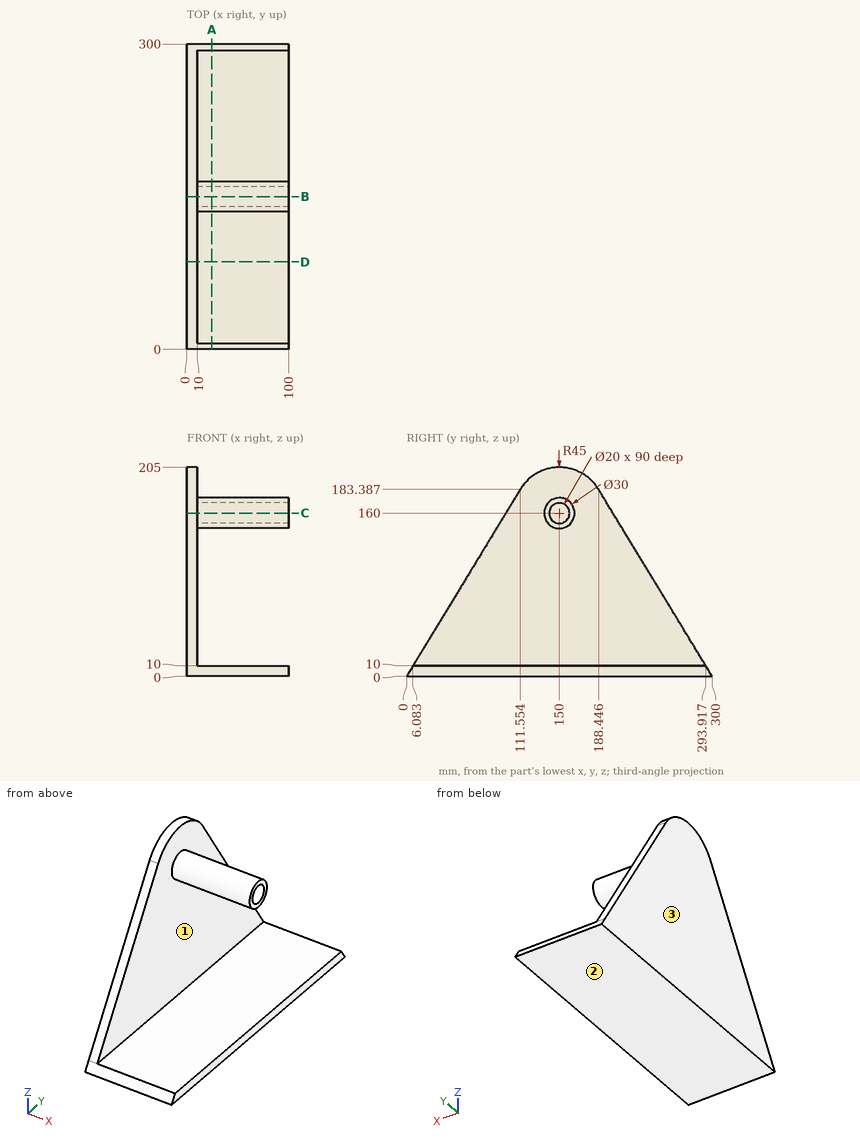
Input: dimensioned drawing with shaded views. Units: mm. Origin: part minimum x, y, z. Coordinates: 2 decimals unless noted, no trailing zeros. Loops run counter-clockwise (first coordinate to the right, second up) from the corner with the lowest first, then second, coordinate; pieces in that order, holes last. Notation, with made-up numbers: (32, 75) -> (39, 75) arc R21 ccw to (39, 112) -> close; hole circle Ø4 at (37, 31). An arc over 180 degrees is marked (long way). One line per item, written item: value. Start each with the question number.
Q1. Line query: line 1 along Z through (x, y) = (53, 150); line 2 along X through (y, z) = (30.5, 28); line 3 along Y through (x, z) = (70.5, 151) (1 decimal). Output: solid intervals per line, ascending.
Q2. Contact query for flat-ended pins moving along their axis: P1, Ø4, axis at x = 21, y = 85.5, coming from the +Z side; P2, Ø1.5, axis at x = 30.5, z = 166.5, coming from the +Y side (1 decimal); P3, Ø1, axis at x = 54.5, z = 156.5, coming from the +Y side. Output: stop coordinate, or through.
Q3. Mould query, pull axis Z, two halves, no side actions, for the marked faces 1, 2 and 3. Classes: pulls with the +Z half, pulls with the -Z half, needs draft (parallel to the pull), parting line crosses it, or undercut.
Q4. Section query A-A, the plane x = 24.5. Return the cut outline in (y, z), and give its area (3 significant figures).
Q5. Section query D-D, the plane y = 86. Return the cut outline in (x, z), and give its area (3 significant figures).
Q6. Section query C-C, the plane z = 160. Return the cut outline in (x, y).
Q7. Section query B-B, the plane y = 150. Return the cut outline in (x, z), and give its area (3 significant figures).
Results:
1. line 1: 0 to 10, 145 to 150, 170 to 175
1. line 2: 0 to 10
1. line 3: 138 to 145.6, 154.4 to 162
2. P1: z = 10
2. P2: y = 163.9
2. P3: y = 164.7
3. face 1: undercut
3. face 2: pulls with the -Z half
3. face 3: needs draft
4. outline: (0, 0) -> (300, 0) -> (293.92, 10) -> (6.08, 10) -> close; circle Ø30 at (150, 160); hole circle Ø20 at (150, 160)
4. area: 3,330 mm^2
5. outline: (0, 0) -> (100, 0) -> (100, 10) -> (10, 10) -> (10, 141.38) -> (0, 141.38) -> close
5. area: 2,310 mm^2
6. outline: (0, 97.33) -> (10, 97.33) -> (10, 135) -> (100, 135) -> (100, 140) -> (10, 140) -> (10, 160) -> (100, 160) -> (100, 165) -> (10, 165) -> (10, 202.67) -> (0, 202.67) -> close
7. outline: (0, 0) -> (100, 0) -> (100, 10) -> (10, 10) -> (10, 145) -> (100, 145) -> (100, 150) -> (10, 150) -> (10, 170) -> (100, 170) -> (100, 175) -> (10, 175) -> (10, 205) -> (0, 205) -> close
7. area: 3,850 mm^2
